The model under review builds one solid part; all positions refer to its coordinate system, in mm. Face numbers are marked on the shaded views. A direction names the side the tool comes from. Give positions to 0.01 mm unless a question says otherwise; leave off trailing zeros. Loops run counter-clockwise (first coordinate to the right, second up) from the corner with the lowest first, then second, coordinate; pieces in that order, holes last. Notation, with made-up numbers: (46.5, -21) - (50.5, -21) arc R22 ccw to (50.5, 4) - close; hole circle Ø5 at (19.5, 57.25). An arc over 180 degrees is marked (long way). Return JSON: item names as keys, results as strings. Group by question number.
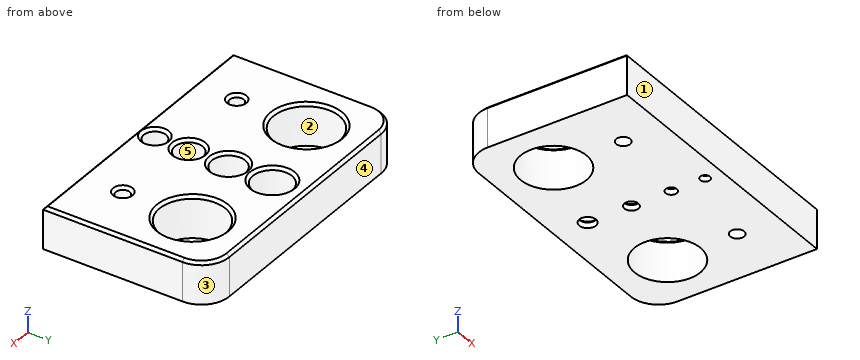
```python
from build123d import *

# Parameters (mm, degrees)
SKETCH_W        = 100
SKETCH_H        = 60
SKETCH_R        = 11.8
SKETCH_R_2      = 2.5
PAD_DEPTH       = 15
FILLET_R        = 10
SKETCH001_R     = 7
SKETCH001_R_2   = 6
SKETCH001_R_3   = 5
SKETCH001_R_4   = 4
POCKET_DEPTH    = 12
SKETCH002_R     = 3
SKETCH002_R_2   = 2.5
SKETCH002_R_3   = 1.75
SKETCH002_R_4   = 2
POCKET001_DEPTH = 5
CHAMFER_SIZE    = 1
CHAMFER001_SIZE = 1


with BuildPart() as part:
    # Sketch → Pad (new body)
    with BuildSketch(Plane.XY):
        Rectangle(SKETCH_W, SKETCH_H)
        with Locations((-30, 10)):
            Circle(SKETCH_R, mode=Mode.SUBTRACT)
        with Locations((30, 10)):
            Circle(SKETCH_R, mode=Mode.SUBTRACT)
        with Locations((-30, -15)):
            Circle(SKETCH_R_2, mode=Mode.SUBTRACT)
        with Locations((30, -15)):
            Circle(SKETCH_R_2, mode=Mode.SUBTRACT)
    extrude(amount=PAD_DEPTH)

    # Fillet
    fillet_edges = [part.edges().sort_by_distance(p)[0] for p in [
        (-50, 30, 7.5),
        (50, 30, 7.5),
    ]]
    fillet(fillet_edges, radius=FILLET_R)

    # Sketch001 → Pocket (cut)
    with BuildSketch(Plane.XY.offset(15)):
        with Locations((0, 18.207773)):
            Circle(SKETCH001_R)
        with Locations((0, 2.49911)):
            Circle(SKETCH001_R_2)
        with Locations((0, -11.781498)):
            Circle(SKETCH001_R_3)
        with Locations((0, -23.920012)):
            Circle(SKETCH001_R_4)
    extrude(amount=-POCKET_DEPTH, mode=Mode.SUBTRACT)

    # Sketch002 → Pocket001 (cut)
    with BuildSketch(Plane.XY.offset(3)):
        with Locations((0, 18.207773)):
            Circle(SKETCH002_R)
        with Locations((0, 2.49911)):
            Circle(SKETCH002_R_2)
        with Locations((0, -23.920012)):
            Circle(SKETCH002_R_3)
        with Locations((0, -11.781498)):
            Circle(SKETCH002_R_4)
    extrude(amount=-POCKET001_DEPTH, mode=Mode.SUBTRACT)

    # Chamfer
    chamfer_edges = [part.edges().sort_by_distance(p)[0] for p in [
        (0, 30, 15),
        (-47.071068, 27.071068, 15),
        (47.071068, 27.071068, 15),
        (-50, -5, 15),
        (50, -5, 15),
        (0, -30, 15),
        (-4, -23.920012, 15),
        (-5, -11.781498, 15),
        (-7, 18.207773, 15),
        (-6, 2.49911, 15),
        (-32.5, -15, 15),
        (-41.8, 10, 15),
        (18.2, 10, 15),
        (27.5, -15, 15),
    ]]
    chamfer(chamfer_edges, length=CHAMFER_SIZE)

    # Chamfer001
    chamfer001_edges = [part.edges().sort_by_distance(p)[0] for p in [
        (-3, 18.207773, 3),
        (-2.5, 2.49911, 3),
        (-2, -11.781498, 3),
        (-1.75, -23.920012, 3),
    ]]
    chamfer(chamfer001_edges, length=CHAMFER001_SIZE)


solid = part.part
```
1) Tool access review of the marked faces 4 and 5: name each direction out of +Z, -Z, +X, -X, +Y, -Y from which nothing blocks a thin tool from reaching the whole face with its end or side.
2) To check wall thickness, follow line 1 (Y direction, x = -30, z = 6); line 2 (Y direction, x = 0, z = 0.6); line 3 (Y direction, x = 0, z = 7). State the ranges of each line that lie inside material, in increasing order.
3) We need section B-B, the plane z = 1. Count the separate pieces of the cut face and the enclosed holes in it, plus the area to 3 significant figures.
4) For pin 1 Ø5.5 at (x, y) = (0, 18.21) entering from -Z; pin 2 Ø8 at (x, y) = (0, 2.5) entering from +Z; pin 3 Ø4 at (x, y) = (-1, -22) entering from +Z; pin 4 Ø11.5 at (x, y) = (0, -11.78) entering from +Z, all flat-tipped, find the tip position at first contact; note any pin that passes through.
5) Draft analysis for pull direction X (two halves, no side actions). For the marked faces 1, 2 and 3, state which applies: +X half, -X half, draft (parallel to the pull), parting line (faces both ways), or undercut.
6) We need section A-A, the plane x = -30. Write out the cut boundary in (y, z), plus the area to 3 significant figures.
Findings:
{
 "1": {"face 4": "+Z, -Z, +X, -X, +Y", "face 5": "+Z"},
 "2": {"line 1": "y = -30 to -17.5, -12.5 to -1.8, 21.8 to 30", "line 2": "y = -30 to -25.67, -22.17 to -13.78, -9.78 to 0, 5 to 15.21, 21.21 to 30", "line 3": "y = -30 to -27.92, -19.92 to -16.78, -6.78 to -3.5, 8.5 to 11.21, 25.21 to 30"},
 "3": {"separate pieces": "1", "enclosed holes": "8", "area": "4,970 mm^2"},
 "4": {"pin 1": "passes through", "pin 2": "stops at z = 3", "pin 3": "stops at z = 14.16", "pin 4": "stops at z = 14.75"},
 "5": {"face 1": "draft", "face 2": "undercut", "face 3": "+X half"},
 "6": {"outline": "(-30, 0) - (-17.5, 0) - (-17.5, 14) - (-18.5, 15) - (-29, 15) - (-30, 14) - close; (-12.5, 0) - (-1.8, 0) - (-1.8, 14) - (-2.8, 15) - (-11.5, 15) - (-12.5, 14) - close; (21.8, 0) - (30, 0) - (30, 14) - (29, 15) - (22.8, 15) - (21.8, 14) - close", "area": "468 mm^2"}
}
